For this review, take the finished solid that the model builds, in its own axes (mm). Give positions to 0.01 mm unless a question says otherwise; leave off trailing zeros. Loops run counter-clockwise (first coordinate to the right, second up) from the corner with the lowest first, then second, coordinate; pieces in that order, holes last.
```python
from build123d import *


with BuildPart() as f1:
    # F0 (on Top) → F1 (revolve)
    with BuildSketch(Plane.XY):
        Polygon((0, -22.373166), (0, 0), (-54.182574, 0), (-59.810659, -22.235475), (-61.148187, -27.519786), (0, -27.519786), align=None)
        Polygon((0, -41.5557), (0, -27.519786), (-61.148187, -27.519786), (-69.370231, -35.74183), (-69.370231, -41.5557), align=None)
        Polygon((0, -47.975048), (0, -41.5557), (-69.370231, -41.5557), (-69.370231, -47.369569), (-61.148187, -55.591614), (0, -55.591614), align=None)
        Polygon((0, -83.111399), (0, -55.591614), (-61.148187, -55.591614), (-59.810659, -60.875925), (-54.182574, -83.111399), align=None)
    revolve(axis=Axis((0, -11.186583, 0), (0, -1, 0)))


solid = f1.part
```
Q1. For probe 1 along Z at (x, y) = (0, -36); probe 2 along X at (y, z) = (-65, 29); probe 3 along X at (y, z) = (-46.5, 32), list the stretches that pass through material, from the lowest coordinate up.
Answers:
probe 1: z = -69.37 to 69.37
probe 2: x = -51.11 to 51.11
probe 3: x = -61.55 to 61.55
Q2. For pin 1 Ø1.5 at (x, y) = (-4, -26) entering from +Z; pin 2 Ø1 at (y, z) = (-19.5, 49) entering from +X; pin 3 Ø2 at (x, y) = (-33, -26.5) entering from -Z; pin 4 Ø6 at (x, z) = (-8, 17.5) entering from +Y, all flat-tipped, find the tip position at first contact; note any pin that passes through.
Answers:
pin 1: stops at z = 60.83
pin 2: stops at x = 33.84
pin 3: stops at z = -51.87
pin 4: stops at y = 0
Q3. Consider section A-A on x = 0. Give the boundary of the cut face in (y, z).
Answers:
outline: (-83.11, -54.18) - (-60.88, -59.81) - (-55.59, -61.15) - (-47.37, -69.37) - (-35.74, -69.37) - (-27.52, -61.15) - (-22.24, -59.81) - (0, -54.18) - (0, 54.18) - (-22.24, 59.81) - (-27.52, 61.15) - (-35.74, 69.37) - (-47.37, 69.37) - (-55.59, 61.15) - (-60.88, 59.81) - (-83.11, 54.18) - close
Q4. Consider section C-C on y = -9.5. Give the boundary of the cut face in (x, z).
Answers:
outline: circle Ø113.17 at (0, 0)
Q5. Consider section D-D on y = -70. Give the boundary of the cut face in (x, z), plus the area to 3 significant figures.
Answers:
outline: circle Ø115 at (0, 0)
area: 10,400 mm2
Q6. Mouldability with a two-part tool opening along Z and no side actions: class faces 1 (the flat face through (-1, 0, -1)), 2 (the conical face through (13.342, -55.192, 60.084)) as +Z half, -Z half, draft (parallel to the pull), parting line (faces both ways), or undercut.
Answers:
face 1: draft
face 2: parting line
Q7. Consider section B-B on z = 0. Give the boundary of the cut face in (x, y), plus the area to 3 significant figures.
Answers:
outline: (-69.37, -47.37) - (-61.15, -55.59) - (-59.81, -60.88) - (-54.18, -83.11) - (54.18, -83.11) - (59.81, -60.88) - (61.15, -55.59) - (69.37, -47.37) - (69.37, -35.74) - (61.15, -27.52) - (59.81, -22.24) - (54.18, 0) - (-54.18, 0) - (-59.81, -22.24) - (-61.15, -27.52) - (-69.37, -35.74) - close
area: 10,100 mm2
